Geometry check sheet. Reference: the model listing, model coordinates, mm. Face numbers are marked on the shaded views. A direction names the side the tool comes from. Coordinates: 2 decimals unless noted, no trailing zeros. Order: outer loops, then holes, each group sorted by start corner. A loop starts at its lowest first (then second) coordinate and runs counter-clockwise, first axis right, second up. Notation, with made-up numbers: M -32.5,74 L 19.5,74 A15 cw 19.5,81 Z; hole C 63.5,-15 d10. An arc over 180 degrees is marked long. One line per item, written item: value. Start each with the question number.
1) Access from +Z, -Z, +X, -X, +Y, -Y to the whole of each face (thin tool, end or side, straight path). Record for the marked faces 1, 2 and 3.
2) Sectioned sample at D-D, the plane x = -107. Enter the section's corners in (y, z), then the cut area to 3 significant figures.
3) Thickness scan on L1, parallel to Y at x = -240, z = 35; L2, parallel to Y at x = -215, z = 35; L3, parallel to X at y = -228.5, z = 24.5. Record the ranges inside material, lowest first. Write a range as from..to.
4) Sectioned sample at A-A, the plane z = 35. Enter the section's corners in (x, y), then the cut area to 3 significant figures.
5) Go/stop test with flat-tipped pins: P1, Ø12, axis at x = -131, z = 53, coming from the +Y side; P2, Ø8, axis at y = -147.5, z = 30.5, coming from the -X side; P3, Ø10, axis at x = -84, z = 31, coming from the -Y side; P4, Ø6, axis at y = -62.5, z = 46.5, coming from the -X side. Record where each tip stops, or that it passes through.
6) Sectioned sample at C-C, the plane y = 75.5. Enter the section's corners in (x, z).
7) Sectioned sample at B-B, the plane x = -221. Enter the section's corners in (y, z).
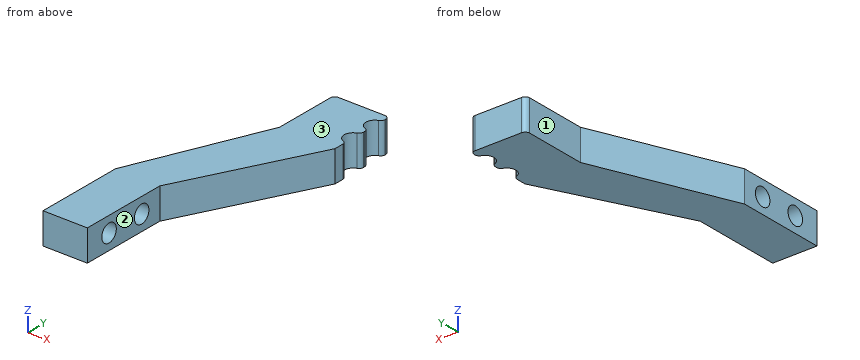
```python
from build123d import *

# Parameters (mm, degrees)
BOSS_EXTRUDE2_DEPTH = 70
SKETCH2_W           = 100
SKETCH2_H           = 200
BOSS_EXTRUDE3_DEPTH = 70
SKETCH3_R           = 20
CUT_EXTRUDE1_DEPTH  = 132
CUT_EXTRUDE2_DEPTH  = 132
CUT_EXTRUDE3_DEPTH  = 132
CUT_EXTRUDE4_DEPTH  = 79
CUT_EXTRUDE6_DEPTH  = 79
CUT_EXTRUDE7_DEPTH  = 79
CUT_EXTRUDE8_DEPTH  = 79


with BuildPart() as part:
    # Sketch1 → Boss-Extrude2 (new body)
    with BuildSketch(Plane.XY):
        Polygon((-137.278106509, 244.304733728), (-12.278106509, 244.304733728), (-12.278106509, -205.695266272), (-262.278106509, -205.695266272), (-137.278106509, 94.304733728), align=None)
    extrude(amount=BOSS_EXTRUDE2_DEPTH)

    # Sketch2 → Boss-Extrude3 (add)
    with BuildSketch(Plane.XY.offset(70)):
        with Locations((-212.278106509, -305.695266272)):
            Rectangle(SKETCH2_W, SKETCH2_H)
    extrude(amount=-BOSS_EXTRUDE3_DEPTH)

    # Sketch3 → Cut-Extrude1 (cut)
    with BuildSketch(Plane(origin=(-162.278106509, 0, 0), x_dir=(0, 0, -1), z_dir=(1, 0, 0))):
        with Locations((-35, -255.695266272)):
            Circle(SKETCH3_R)
        with Locations((-35, -345.695266272)):
            Circle(SKETCH3_R)
    extrude(amount=-CUT_EXTRUDE1_DEPTH, mode=Mode.SUBTRACT)

    # Sketch5 → Cut-Extrude2 (cut)
    with BuildSketch(Plane.XY.offset(70)):
        Polygon((-12.278106509, 94.304733728), (-12.278106509, -205.695266272), (-162.278106509, -205.695266272), align=None)
    extrude(amount=-CUT_EXTRUDE2_DEPTH, mode=Mode.SUBTRACT)

    # Sketch6 → Cut-Extrude3 (cut)
    with BuildSketch(Plane.XY.offset(70)):
        with BuildLine():
            Line((-12.278106509, 224.304733728), (-12.278106509, 204.304733728))
            Line((-12.278106509, 204.304733728), (-12.278106509, 184.304733728))
            ThreePointArc((-12.278106509, 184.304733728), (-32.278106509, 204.304733728), (-12.278106509, 224.304733728))
        make_face()
        with BuildLine():
            Line((-12.278106509, 144.304733728), (-12.278106509, 124.304733728))
            ThreePointArc((-12.278106509, 124.304733728), (-32.278106509, 144.304733728), (-12.278106509, 164.304733728))
            Line((-12.278106509, 164.304733728), (-12.278106509, 144.304733728))
        make_face()
    extrude(amount=-CUT_EXTRUDE3_DEPTH, mode=Mode.SUBTRACT)

    # Sketch9 → Cut-Extrude4 (cut)
    with BuildSketch(Plane.XY.offset(70)):
        with BuildLine():
            Line((-127.278106509, 244.304733728), (-137.278106509, 244.304733728))
            Line((-137.278106509, 244.304733728), (-137.278106509, 234.304733728))
            ThreePointArc((-137.278106509, 234.304733728), (-134.349174321, 241.37580154), (-127.278106509, 244.304733728))
        make_face()
    extrude(amount=-CUT_EXTRUDE4_DEPTH, mode=Mode.SUBTRACT)

    # Sketch11 → Cut-Extrude6 (cut)
    with BuildSketch(Plane.XY.offset(70)):
        with BuildLine():
            Line((-12.278106509, 232.589004975), (-12.278106509, 224.304733728))
            Line((-12.278106509, 224.304733728), (-18.944773176, 223.160914559))
            ThreePointArc((-18.944773176, 223.160914559), (-14.1131407, 226.815502283), (-12.278106509, 232.589004975))
        make_face()
    extrude(amount=-CUT_EXTRUDE6_DEPTH, mode=Mode.SUBTRACT)

    # Sketch12 → Cut-Extrude7 (cut)
    with BuildSketch(Plane.XY.offset(70)):
        with BuildLine():
            Line((-18.944773176, 125.448552896), (-12.278106509, 124.304733728))
            Line((-12.278106509, 124.304733728), (-12.278106509, 116.02046248))
            ThreePointArc((-12.278106509, 116.02046248), (-14.1131407, 121.793965172), (-18.944773176, 125.448552896))
        make_face()
        with BuildLine():
            Line((-18.944773176, 185.448552896), (-12.278106509, 184.304733728))
            Line((-12.278106509, 184.304733728), (-12.278106509, 176.02046248))
            ThreePointArc((-12.278106509, 176.02046248), (-14.1131407, 181.793965172), (-18.944773176, 185.448552896))
        make_face()
        with BuildLine():
            Line((-18.944773176, 163.160914559), (-12.278106509, 164.304733728))
            Line((-12.278106509, 164.304733728), (-12.278106509, 172.589004975))
            ThreePointArc((-12.278106509, 172.589004975), (-14.1131407, 166.815502283), (-18.944773176, 163.160914559))
        make_face()
    extrude(amount=-CUT_EXTRUDE7_DEPTH, mode=Mode.SUBTRACT)

    # Sketch13 → Cut-Extrude8 (cut)
    with BuildSketch(Plane.XY.offset(70)):
        with BuildLine():
            Line((-22.278106509, 244.304733728), (-12.278106509, 244.304733728))
            Line((-12.278106509, 244.304733728), (-12.278106509, 234.304733728))
            ThreePointArc((-12.278106509, 234.304733728), (-15.207038697, 241.37580154), (-22.278106509, 244.304733728))
        make_face()
    extrude(amount=-CUT_EXTRUDE8_DEPTH, mode=Mode.SUBTRACT)


solid = part.part
```
Final values:
1. face 1: +Z, -Z, -X, +Y
1. face 2: +Z, -Z, +X, -Y
1. face 3: +Z, +X, -X, +Y, -Y
2. outline: M -95.14,0 L 244.3,0 L 244.3,70 L -95.14,70 Z
2. area: 23,800 mm^2
3. L1: y = -405.7..-365.7, -325.7..-275.7, -235.7..-152.23
3. L2: y = -405.7..-365.7, -325.7..-275.7, -235.7..-92.23
3. L3: x = -262.28..-162.28
4. outline: M -262.28,-405.7 L -162.28,-405.7 L -162.28,-365.7 L -262.28,-365.7 Z; M -262.28,-325.7 L -162.28,-325.7 L -162.28,-275.7 L -262.28,-275.7 Z; M -262.28,-235.7 L -162.28,-235.7 L -162.28,-205.7 L -12.28,94.3 L -12.28,116.02 A10 ccw -18.94,125.45 A20 cw -18.94,163.16 A10 ccw -12.28,172.59 L -12.28,176.02 A10 ccw -18.94,185.45 A20 cw -18.94,223.16 A10 ccw -12.28,232.59 L -12.28,234.3 A10 ccw -22.28,244.3 L -127.28,244.3 A10 ccw -137.28,234.3 L -137.28,94.3 L -262.28,-205.7 Z
4. area: 63,200 mm^2
5. P1: stops at y = 244.3
5. P2: stops at x = -239.7
5. P3: stops at y = -59.14
5. P4: stops at x = -203.86
6. outline: M -145.11,0 L -21.68,0 L -21.68,70 L -145.11,70 Z
7. outline: M -405.7,0 L -106.63,0 L -106.63,70 L -405.7,70 Z; hole C -345.7,35 d40; hole C -255.7,35 d40
